```python
from build123d import *

# Parameters (mm, degrees)
PAD_DEPTH       = 15
PAD001_DEPTH    = 11
SKETCH002_R     = 4.02
HOLE_DEPTH      = 25
POCKET_DEPTH    = 21
POCKET001_DEPTH = 6.7


with BuildPart() as body:
    # Sketch → Pad (new body)
    with BuildSketch(Plane.XZ):
        Polygon((30, 4.667262), (11.667262, 23), (0, 11.332738), (0, 0), (30, 0), align=None)
    extrude(amount=PAD_DEPTH)

    # Sketch001 → Pad001 (join)
    with BuildSketch(Plane.XY):
        with BuildLine():
            ThreePointArc((0, -27.02), (4.02, -23), (0, -18.98))
            Line((0, -18.98), (0, -15))
            Line((0, -15), (15.491933, -15))
            ThreePointArc((15.491933, -15), (12.329656, -16.55051), (11.61895, -20))
            ThreePointArc((0, -35), (9.486833, -30.348469), (11.61895, -20))
            Line((0, -35), (0, -27.02))
        make_face()
    extrude(amount=PAD001_DEPTH)

    # Sketch002 (on DatumPlane) → Hole (cut)
    with BuildSketch(Plane(origin=(17.333631, 0, 17.333631), x_dir=(-0.707107, 0, 0.707107), z_dir=(0.707107, 0, 0.707107))):
        with Locations((-1.486544, 0)):
            Circle(SKETCH002_R)
    extrude(amount=-HOLE_DEPTH, mode=Mode.SUBTRACT)

    # Sketch003 (on DatumPlane) → Pocket (cut)
    with BuildSketch(Plane(origin=(8.131728, 0, 19.464466), x_dir=(0, 1, 0), z_dir=(0.707107, 0, 0.707107))):
        Polygon((-7.794229, -9.5), (-3.897114, -16.25), (3.897114, -16.25), (7.794229, -9.5), (3.897114, -2.75), (-3.897114, -2.75), align=None)
    extrude(amount=-POCKET_DEPTH, mode=Mode.SUBTRACT)

    # Sketch004 (on Face13 of Pocket) → Pocket001 (cut)
    with BuildSketch(Plane(origin=(0, 0, 11), x_dir=(-1, 0, 0), z_dir=(0, 0, 1))):
        Polygon((-3.897114, 29.75), (-7.794229, 23), (-3.897114, 16.25), (3.897114, 16.25), (7.794229, 23), (3.897114, 29.75), align=None)
    extrude(amount=-POCKET001_DEPTH, mode=Mode.SUBTRACT)


with BuildPart() as part_mirroring:
    # Part__Mirroring: instance of Body
    add(body.part.mirror(Plane(origin=(0, 0, 0), x_dir=(1, 0, 0), z_dir=(0, 1, 0))))


with BuildPart() as part_mirroring001:
    # Part__Mirroring001: instance of Part__Mirroring
    add(part_mirroring.part.mirror(Plane(origin=(0, 0, 0), x_dir=(0, -1, 0), z_dir=(1, 0, 0))))


with BuildPart() as fusion:
    # Part__Mirroring002: instance of Body
    add(body.part.mirror(Plane(origin=(0, 0, 0), x_dir=(0, -1, 0), z_dir=(1, 0, 0))))

    # Fusion: union Part__Mirroring001, Part__Mirroring, Body
    add(part_mirroring001.part)
    add(part_mirroring.part)
    add(body.part)


solid = fusion.part
```
CAD build for the part. Positions are in the model's coordinates, mm. A direction names the side the tool comes from. Give positions to 0.01 mm unless a question says otherwise; leave off trailing zeros. Loops run counter-clockwise (first coordinate to the right, second up) from the corner with the lowest first, then second, coordinate; pieces in that order, holes last. Notation, with made-up numbers: (-34.75, 63.25) - (-24.75, 63.25) arc R15 ccw to (-24.75, 81.25) - close; hole circle Ø7 at (-38, 85). An arc over 180 degrees is marked (long way). Put each result on its own line as item: value.
Q1. Slice it at C-C (y = -3). Give the cut face in (x, z).
Filled in:
outline: (-30, 0) - (-11.65, 0) - (-19.62, 7.97) - (-16.74, 10.85) - (-20.28, 14.39) - (-30, 4.67) - close; (-16.49, 18.17) - (-12.96, 14.64) - (-10.08, 17.52) - (0, 7.44) - (10.08, 17.52) - (12.96, 14.64) - (16.49, 18.17) - (11.67, 23) - (0, 11.33) - (-11.67, 23) - close; (11.65, 0) - (30, 0) - (30, 4.67) - (20.28, 14.39) - (16.74, 10.85) - (19.62, 7.97) - close
Q2. Slice it at B-B (y = -12.5). Give the cut face in (x, z).
Filled in:
outline: (-30, 0) - (30, 0) - (30, 4.67) - (11.67, 23) - (0, 11.33) - (-11.67, 23) - (-30, 4.67) - close
Q3. Tool access for faces 4 (the face through (3, 26, 4.3)), 5 (the face through (-5.92, -0.21, 17.25)), 6 (the face through (12.334, 5.873, 5.526)), 7 (the face through (-7, -15, 12)): list every direction of +Z, -Z, +X, -X, +Y, -Y with a clear straight run to the whole face (end or side of a thin tool).
Filled in:
face 4: +Z
face 5: +Z, +Y, -Y
face 6: none
face 7: +Z, -Y
Q4. Mould opens along X. For faces 1 (the face through (7, -25, 11)), 2 (the face through (12.36, -16.51, 5.42)), 3 (the face through (0, -16.25, 8)) say: pulls with the +X half, pulls with the -X half, needs draft (parallel to the pull), parting line crosses it, or undercut.
Filled in:
face 1: needs draft
face 2: pulls with the +X half
face 3: undercut
Q5. Slice it at A-A (x = -1). Give the cut face in (y, z), plus the area to 3 significant figures.
Filled in:
outline: (-34.96, 0) - (-26.89, 0) - (-26.89, 4.3) - (-29.75, 4.3) - (-29.75, 11) - (-34.96, 11) - close; (-19.11, 0) - (-7.34, 0) - (-3.9, 8.44) - (3.9, 8.44) - (7.34, 0) - (19.11, 0) - (19.11, 4.3) - (16.25, 4.3) - (16.25, 11) - (15, 11) - (15, 12.33) - (-15, 12.33) - (-15, 11) - (-16.25, 11) - (-16.25, 4.3) - (-19.11, 4.3) - close; (26.89, 0) - (34.96, 0) - (34.96, 11) - (29.75, 11) - (29.75, 4.3) - (26.89, 4.3) - close
area: 466 mm²
Q6. Flat gauge pins, fed straight in: pin 1 (2 mm diameter, centred on y = 20, z = 10, fed in from +X); pin 2 (10 mm diameter, centred on x = -21, z = 19, fed in from -Y); pin 3 (4 mm diameter, centred on x = -1.5, y = -23, fed in from +Z) (3 decimals); pin 4 (4 mm diameter, centred on y = 27.5, z = 7, fed in from -X). Where does each tip first touch, or does it go through?
Filled in:
pin 1: stops at x = 11.83
pin 2: stops at y = -15
pin 3: passes through
pin 4: stops at x = -11.74
Q7. Probe line 1 along X through (y, z) = (-23, 3.35); line 2 along Y through (x, z) = (6, 8.5); line 3 along Y through (x, z) = (27.5, 2.75). List the from-to ranges inside material, lowest first.
Filled in:
line 1: x = -12 to -4.02, 4.02 to 12
line 2: y = -33.39 to -26.11, -19.89 to -5.92, 5.92 to 19.89, 26.11 to 33.39
line 3: y = -15 to 15
Q8. Slice it at D-D (y = 21). Give the cut face in (x, z), plus the area to 3 significant figures.
Filled in:
outline: (-11.83, 0) - (-3.49, 0) - (-3.49, 4.3) - (-6.64, 4.3) - (-6.64, 11) - (-11.83, 11) - close; (3.49, 0) - (11.83, 0) - (11.83, 11) - (6.64, 11) - (6.64, 4.3) - (3.49, 4.3) - close
area: 141 mm²
